Print and shaded views of the part. All mm, measured from the part's lowest x, y and z. Give positions to 0.01 mm unless a question says otherwise; leave off trailing zeros. Write each loop counter-clockwise with the first axis right and the second up, starting at its lowest first coordinate (ties: lowest second). Pieces come first, ordered by that corner, then holes.
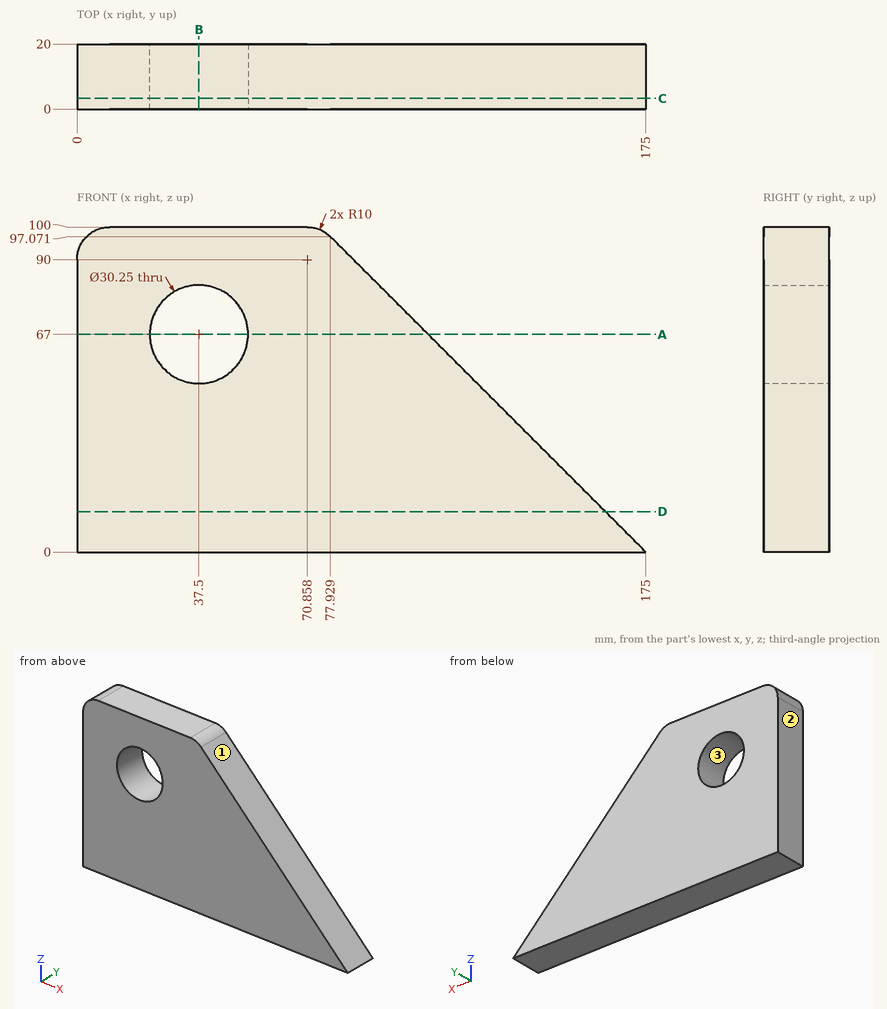
1. Saw through at A-A on z = 67. Give the cut face in (x, y) (3 decimals), plus the area to 4 significant figures.
2. Saw through at D-D on z = 12.5. Give the cut face in (x, y).
3. Mould opens along X. For the marked faces 1, 2 and 3 say: pulls with the +X half, pulls with the -X half, needs draft (parallel to the pull), parting line crosses it, or undercut.
4. Drop flat-ended pins along their axis: pin 1 (5 mm diameter, centred on y = 8.5, z = 87.5, fed in from +X); pin 2 (1.5 mm diameter, centred on x = 131.5, y = 16.5, fed in from +Z); pin 3 (8 mm diameter, centred on y = 3.5, z = 42, fed in from +X). Give the stop position or say it passes through.
5. Drill centre lines: line 1 along Z through (x, y) = (37.5, 9.25) (3 decimals); line 2 along Z through (x, y) = (42.5, 8.75) (1 decimal); line 3 along X through (y, z) = (7.5, 71). Where is each one in solid material? Low to high.
6. Saw through at C-C on y = 3.25. Give the cut face in (x, z) (3 decimals).
7. Saw through at B-B on x = 37.5. Give the cut face in (y, z) (3 decimals).
Outcome:
1. outline: (0, 0) - (22.375, 0) - (22.375, 20) - (0, 20) - close; (52.625, 0) - (108, 0) - (108, 20) - (52.625, 20) - close
1. area: 1,555 mm2
2. outline: (0, 0) - (162.5, 0) - (162.5, 20) - (0, 20) - close
3. face 1: pulls with the +X half
3. face 2: pulls with the -X half
3. face 3: undercut
4. pin 1: stops at x = 90
4. pin 2: stops at z = 44.25
4. pin 3: stops at x = 137
5. line 1: z = 0 to 51.875, 82.125 to 100
5. line 2: z = 0 to 52.7, 81.3 to 100
5. line 3: x = 0 to 22.91, 52.09 to 104
6. outline: (0, 0) - (175, 0) - (77.929, 97.071) arc R10 ccw to (70.858, 100) - (10, 100) arc R10 ccw to (0, 90) - close; hole circle Ø30.25 at (37.5, 67)
7. outline: (0, 0) - (20, 0) - (20, 51.875) - (0, 51.875) - close; (0, 82.125) - (20, 82.125) - (20, 100) - (0, 100) - close
